Verification items for the finished model (mm, model axes). Round coordinates to 2 decimals unless told otherwise and drop trailing zeros. Answer as a JSON object with one key per item and string values. Group by question number.
(1) Draft check along Z on faces 1 (the face through (-57, -25.4, 43)), 2 (the face through (-57.14, -8.91, 47.45)), 3 (the face through (-57, -13, 28.505)), 4 (the face through (-55.8, -16.1, 47.7)). Enter one of: released by +Z, released by -Z, zero draft, split by the parting line, or undercut.
(2) Gauge pin test, flat end, axial feed: pin 1 Ø2 at (x, z) = (-62.5, 55.5) entering from +Y. Record the tip position at first contact, or that the pin passes through.
(3) Scan lines: L1, parallel to Z at x = -56.25, y = -15.5; L2, parallel to Z at x = -58, y = -11.5. Record each from-to range of solid material in increasing order. Write a range as from..to.
```python
from build123d import *

# Parameters (mm, degrees)
F0_W           = 23.6548669636
F0_H           = 35.3559218347
F1_DEPTH       = 25.4
F3_D           = 2.5781
F3_DEPTH       = 15.8496
F3_CSINK_D     = 7.1374
F3_CSINK_ANGLE = 82
F3_TIP         = 0.774539381


with BuildPart() as f1:
    # F0 (on Front) → F1 (new body)
    with BuildSketch(Plane.XZ):
        with Locations((-57.1659114212, 46.1829993874)):
            Rectangle(F0_W, F0_H)
    extrude(amount=F1_DEPTH)

    # F3
    with Locations(Plane.XZ.offset(25.4)):
        with Locations((-57.0883825421, 47.6693250239)):
            CounterSinkHole(F3_D / 2, F3_CSINK_D / 2, depth=F3_DEPTH, counter_sink_angle=F3_CSINK_ANGLE)
            with Locations((0, 0, -(F3_DEPTH + F3_TIP / 2))):  # 118° drill point
                Cone(0, F3_D / 2, F3_TIP, mode=Mode.SUBTRACT)


solid = f1.part
```
Computed values:
{
 "1": {"face 1": "zero draft", "face 2": "undercut", "face 3": "released by -Z", "face 4": "undercut"},
 "2": {"pin 1": "y = 0"},
 "3": {"L1": "28.51..46.69, 48.65..63.86", "L2": "28.51..46.76, 48.58..63.86"}
}
